Study the drawing (mm; zero at the part's minimum x, y, z) and answer. A direction names the side the tool comes from. Coordinates: 2 decimals unless noted, no trailing zeros. Order: outer loops, then holes, each group sorted by start corner. A loop starts at its lowest first (then second) coordinate and runs counter-clockwise, first axis right, second up.
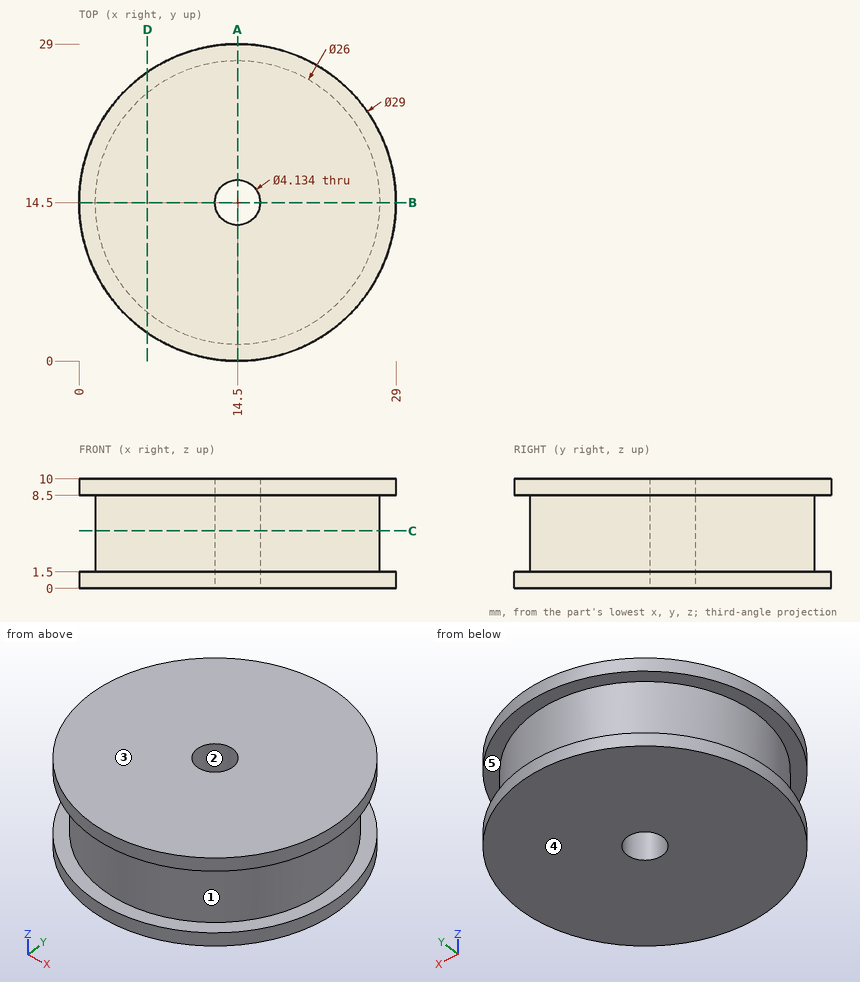
1) Which of the six approach directions +Z, -Z, +X, -X, +Y, -Y give full straight-line access (tool end or side, diameter ignored) to the marked faces 4 and 5?
A:
face 4: -Z, +X, -X, +Y, -Y
face 5: none
2) Flat-ended cylindrical pins translate along their axes: pin 1 Ø5 at (x, z) = (11.5, 5) entering from -Y; pin 2 Ø6 at (x, z) = (21, 3.5) entering from -Y; pin 3 Ø3.5 at (x, y) = (14.5, 14.5) entering from -Z (3 decimals); pin 4 Ø1 at (x, z) = (10, 2.5) entering from -Y. Find the tip coordinate at first contact, or state that the pin passes through.
A:
pin 1: stops at y = 1.51
pin 2: stops at y = 0.64
pin 3: passes through
pin 4: stops at y = 2.13
3) A cutting plane is placed at D-D, the plane x = 6.25. Determine the outline of the cut face in (y, z), and give its area (3 significant figures).
A:
outline: (2.58, 0) - (26.42, 0) - (26.42, 1.5) - (24.55, 1.5) - (24.55, 8.5) - (26.42, 8.5) - (26.42, 10) - (2.58, 10) - (2.58, 8.5) - (4.45, 8.5) - (4.45, 1.5) - (2.58, 1.5) - close
area: 212 mm2
4) A cutting plane is placed at C-C, the plane z = 5.25. Determine the outline of the cut face in (x, y), and give its area (3 significant figures).
A:
outline: circle Ø26 at (14.5, 14.5); hole circle Ø4.13 at (14.5, 14.5)
area: 518 mm2
5) Determine the mould class of the marked faces 1, 2 and 3 for opening direction X: pulls with the +X half, pulls with the -X half, needs draft (parallel to the pull), parting line crosses it, or undercut.
A:
face 1: parting line crosses it
face 2: undercut
face 3: needs draft
6) A cutting plane is placed at A-A, the plane x = 14.5. Determine the outline of the cut face in (y, z), and give its area (3 significant figures).
A:
outline: (0, 0) - (12.43, 0) - (12.43, 10) - (0, 10) - (0, 8.5) - (1.5, 8.5) - (1.5, 1.5) - (0, 1.5) - close; (16.57, 0) - (29, 0) - (29, 1.5) - (27.5, 1.5) - (27.5, 8.5) - (29, 8.5) - (29, 10) - (16.57, 10) - close
area: 228 mm2
7) Straight lines are drawn through the part: line 1 (Y direction, x = 14.5, z = 3.25); line 2 (Y direction, x = 16.25, z = 2.75); line 3 (X direction, y = 7.25, z = 3.5). For each, find the intervals that lie inside material, in ascending order.
A:
line 1: y = 1.5 to 12.43, 16.57 to 27.5
line 2: y = 1.62 to 13.4, 15.6 to 27.38
line 3: x = 3.71 to 25.29
